Geometry: final body of the model. Coordinates: model frame, mm. Coordinates: 2 decimals unless noted, no trailing zeros. Order: outer loops, then holes, each group sorted by start corner. A loop starts at its lowest first (then second) coordinate and runs counter-clockwise, first axis right, second up. Notation, with made-up numbers: (57, -13.5) - (99, -13.5) arc R32 cw to (99, 12.5) - close; hole circle Ø1 at (68, 59.25). An arc over 180 degrees is marked (long way). Use a Markdown table: item, result. Add a question column.
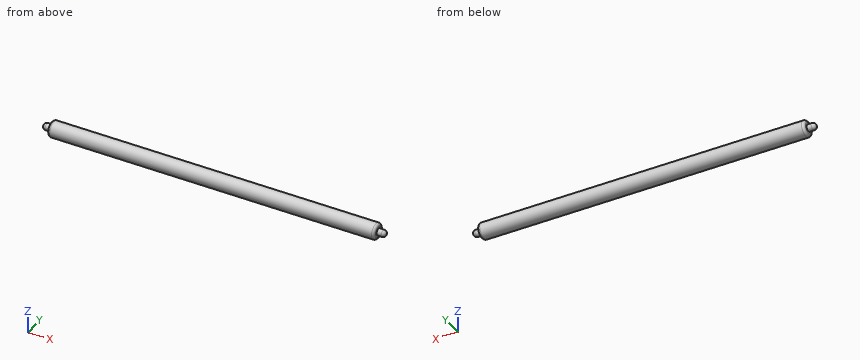
```python
from build123d import *

# Parameters (mm, degrees)
ESBO_O1_R                = 9.25
RESSALTO_EXTRUS_O1_DEPTH = 385
ESBO_O2_R                = 4
RESSALTO_EXTRUS_O2_DEPTH = 9.5
FILETE1_R                = 3
ESBO_O3_R                = 4
RESSALTO_EXTRUS_O3_DEPTH = 9.5
FILETE2_R                = 4


with BuildPart() as part:
    # Esboço1 → Ressalto-extrusão1 (new body)
    with BuildSketch(Plane(origin=(0, 0, 0), x_dir=(0, 0, -1), z_dir=(1, 0, 0))):
        Circle(ESBO_O1_R)
    extrude(amount=RESSALTO_EXTRUS_O1_DEPTH)

    # Esboço2 → Ressalto-extrusão2 (add)
    with BuildSketch(Plane.ZY):
        Circle(ESBO_O2_R)
    extrude(amount=RESSALTO_EXTRUS_O2_DEPTH)

    # Filete1
    filete1_edges = [part.edges().sort_by_distance(p)[0] for p in [
        (0, 0, 9.25),
        (385, 0, 9.25),
    ]]
    fillet(filete1_edges, radius=FILETE1_R)

    # Esboço3 → Ressalto-extrusão3 (add)
    with BuildSketch(Plane(origin=(385, 0, 0), x_dir=(0, 0, -1), z_dir=(1, 0, 0))):
        Circle(ESBO_O3_R)
    extrude(amount=RESSALTO_EXTRUS_O3_DEPTH)

    # Filete2
    filete2_edges = [part.edges().sort_by_distance(p)[0] for p in [
        (394.5, 0, 4),
        (-9.5, 0, -4),
    ]]
    fillet(filete2_edges, radius=FILETE2_R)


solid = part.part
```
1) Section query A-A (z = 0). Return the cut outline in (x, y).
2) Section query C-C (x = 245). Return the cut outline in (y, z), and give its area (3 significant figures).
3) Line query: line 1 (X direction, y = 0.5, z = -0.25); line 2 (Z direction, x = 60, y = 0.75); line 3 (X direction, y = -4, z = -4.25). Output: solid intervals per line, ascending. Write a range as from..to.
4) First-contact query: pin 1 (1 mm diameter, centred on x = 261.5, y = 4.5, fed in from +Z); pin 2 (3 mm diameter, centred on x = 54, y = 2, fed in from +Z); pin 3 (4 mm diameter, centred on x = 111, y = 5.5, fed in from +Z). Flat tips, straight axial feed; report the tip coordinate or a pass-through.
From the geometry:
| question | item | result |
|---|---|---|
| 1 | outline | (-5.5, -4) - (0, -4) - (0, -6.25) arc R3 ccw to (3, -9.25) - (382, -9.25) arc R3 ccw to (385, -6.25) - (385, -4) - (390.5, -4) arc R4 ccw to (390.5, 4) - (385, 4) - (385, 6.25) arc R3 ccw to (382, 9.25) - (3, 9.25) arc R3 ccw to (0, 6.25) - (0, 4) - (-5.5, 4) arc R4 ccw to start |
| 2 | outline | circle Ø18.5 at (0, 0) |
| 2 | area | 269 mm^2 |
| 3 | line 1 | x = -9.46..394.46 |
| 3 | line 2 | z = -9.22..9.22 |
| 3 | line 3 | x = 0..385 |
| 4 | pin 1 | stops at z = 8.34 |
| 4 | pin 2 | stops at z = 9.24 |
| 4 | pin 3 | stops at z = 8.56 |
